Source: CAD feature listing. Evaluate the final solid. Frame: model axes, mm. A direction names the side the tool comes from. Coordinates: 2 decimals unless noted, no trailing zeros. Write each loop counter-clockwise with the first axis right and the second up, starting at its lowest first coordinate (ties: lowest second). Pieces come first, ordered by that corner, then holes. Notation, with made-up numbers: M 87,-1 L 104,-1 A19 ccw 104,12 Z; hole C 79,-3.75 d7. An arc over 180 degrees is marked long. One line per item, written item: value. Start each with the question number.
Item 1: Pin query (flat end, axial travel): P1, Ø3, axis at x = 0, z = 0, coming from the +Y side; P2, Ø2, axis at x = 9.5, z = 2, coming from the +Y side; P3, Ø1.5, axis at y = 1.5, z = -1, coming from the -X side; P4, Ø4, axis at x = -0.5, z = 0, coming from the +Y side. Return the tip coordinate at first contact, or that it passes through.
Item 2: Set-up query: faces 1 (the flat face through (2, 3.9, 2)), 2 (the flat face through (-1, 1, 1)), 3 (the cylindrical face through (-0.5, 2.7, 2.4)). Return all of +Z, -Z, +X, -X, +Y, -Y with unobstructed straight access to the full face (end or side cutting, diameter ignored); none if empty.
Item 3: Cut plane A-A, the plane y = 0.8. State how many separate pieces and enclosed holes the cut face has, then the cut area to 3 significant figures.
Item 4: Cut plane C-C, the plane z = 1.75. Output: boundary loops of the cut face in (x, y).
Item 5: Cut plane B-B, the plane x = 4.5. Output: boundary loops of the cut face in (y, z), then the cut area to 3 significant figures.
Item 6: Ray query, L1, parallel to Z at x = 0, y = 1.2; L2, parallel to Z at x = 15.2, y = 0.6; L3, parallel to X at y = 2.3, z = 0. Return the intervals inside material, ascending. Write a range as from..to.
Item 7: Mould query, pull axis X, two halves, no side actions, for faces 4 (the flat face through (10, 1.4, 1)), 5 (the flat face through (1, 1.5, -1)), 6 (the cylindrical face through (17.2, 0.7, 0)). Classes: released by +X, released by -X, zero draft, split by the parting line, or undercut.
```python
from build123d import *

# Parameters (mm, degrees)
SKETCH1_R           = 0.5
BOSS_EXTRUDE1_DEPTH = 1.4
SKETCH2_R           = 2.35
CUT_EXTRUDE1_DEPTH  = 1
SKETCH3_R           = 3.5
SKETCH3_R_2         = 2.45
BOSS_EXTRUDE2_DEPTH = 2.5
SKETCH4_R           = 1.2
CUT_EXTRUDE2_DEPTH  = 2.4
SKETCH5_R           = 2.45
SKETCH5_R_2         = 1.2
BOSS_EXTRUDE3_DEPTH = 0.1
SKETCH6_W           = 35.735260114
SKETCH6_H           = 17.672039004
CUT_EXTRUDE4_DEPTH  = 4.9
CUT_EXTRUDE5_DEPTH  = 4.9


with BuildPart() as part:
    # Sketch1 → Boss-Extrude1 (new body)
    with BuildSketch(Plane(origin=(0, 0, 0), x_dir=(1, 0, 0), z_dir=(0, 1, 0))):
        with BuildLine():
            Line((-15.2, 2), (-2, 2.95))
            Line((-2, 2.95), (-2, 6.35))
            ThreePointArc((-2, 6.35), (0, 8.35), (2, 6.35))
            Line((2, 6.35), (2, 3.5))
            Line((2, 3.5), (15.2, 2))
            ThreePointArc((15.2, 2), (17.2, 0), (15.2, -2))
            Line((15.2, -2), (2, -3.5))
            Line((2, -3.5), (2, -6.35))
            ThreePointArc((2, -6.35), (0, -8.35), (-2, -6.35))
            Line((-2, -6.35), (-2, -2.95))
            Line((-2, -2.95), (-15.2, -2))
            ThreePointArc((-15.2, -2), (-17.2, 0), (-15.2, 2))
        make_face()
        with Locations((0, 6.35)):
            Circle(SKETCH1_R, mode=Mode.SUBTRACT)
        with Locations((0, 4.55)):
            Circle(SKETCH1_R, mode=Mode.SUBTRACT)
        with Locations((0, -4.55)):
            Circle(SKETCH1_R, mode=Mode.SUBTRACT)
        with Locations((0, -6.35)):
            Circle(SKETCH1_R, mode=Mode.SUBTRACT)
        with Locations((-15.2, 0)):
            Circle(SKETCH1_R, mode=Mode.SUBTRACT)
        with Locations((15.2, 0)):
            Circle(SKETCH1_R, mode=Mode.SUBTRACT)
        with Locations((-13.4, 0)):
            Circle(SKETCH1_R, mode=Mode.SUBTRACT)
        with Locations((-11.6, 0)):
            Circle(SKETCH1_R, mode=Mode.SUBTRACT)
        with Locations((-9.8, 0)):
            Circle(SKETCH1_R, mode=Mode.SUBTRACT)
        with Locations((-8, 0)):
            Circle(SKETCH1_R, mode=Mode.SUBTRACT)
        with Locations((-6.2, 0)):
            Circle(SKETCH1_R, mode=Mode.SUBTRACT)
        with Locations((-4.4, 0)):
            Circle(SKETCH1_R, mode=Mode.SUBTRACT)
        with Locations((13.4, 0)):
            Circle(SKETCH1_R, mode=Mode.SUBTRACT)
        with Locations((11.6, 0)):
            Circle(SKETCH1_R, mode=Mode.SUBTRACT)
        with Locations((9.8, 0)):
            Circle(SKETCH1_R, mode=Mode.SUBTRACT)
        with Locations((8, 0)):
            Circle(SKETCH1_R, mode=Mode.SUBTRACT)
        with Locations((6.2, 0)):
            Circle(SKETCH1_R, mode=Mode.SUBTRACT)
        with Locations((4.4, 0)):
            Circle(SKETCH1_R, mode=Mode.SUBTRACT)
    extrude(amount=BOSS_EXTRUDE1_DEPTH)

    # Sketch2 → Cut-Extrude1 (cut)
    with BuildSketch(Plane.XZ):
        Circle(SKETCH2_R)
    extrude(amount=-CUT_EXTRUDE1_DEPTH, mode=Mode.SUBTRACT)

    # Sketch3 → Boss-Extrude2 (add)
    with BuildSketch(Plane(origin=(0, 1.4, 0), x_dir=(1, 0, 0), z_dir=(0, 1, 0))):
        Circle(SKETCH3_R)
        Circle(SKETCH3_R_2, mode=Mode.SUBTRACT)
    extrude(amount=BOSS_EXTRUDE2_DEPTH)

    # Sketch4 → Cut-Extrude2 (cut, through all)
    with BuildSketch(Plane(origin=(0, 1.4, 0), x_dir=(1, 0, 0), z_dir=(0, 1, 0))):
        Circle(SKETCH4_R)
    extrude(amount=-CUT_EXTRUDE2_DEPTH, mode=Mode.SUBTRACT)

    # Sketch5 → Boss-Extrude3 (add)
    with BuildSketch(Plane(origin=(0, 1.4, 0), x_dir=(1, 0, 0), z_dir=(0, 1, 0))):
        Circle(SKETCH5_R)
        Circle(SKETCH5_R_2, mode=Mode.SUBTRACT)
    extrude(amount=BOSS_EXTRUDE3_DEPTH)

    # Sketch6 → Cut-Extrude4 (cut, through all)
    with BuildSketch(Plane.XZ):
        Rectangle(SKETCH6_W, SKETCH6_H)
        with BuildLine():
            Line((-1.868584713, -2.959457918), (-15.2, -2))
            ThreePointArc((-15.2, -2), (-17.2, 0), (-15.2, 2))
            Line((-15.2, 2), (-1.868584713, 2.959457918))
            ThreePointArc((-1.868584713, 2.959457918), (0, 3.5), (1.868584713, 2.959457918))
            Line((1.868584713, 2.959457918), (15.2, 2))
            ThreePointArc((15.2, 2), (17.2, 0), (15.2, -2))
            Line((15.2, -2), (1.868584713, -2.959457918))
            ThreePointArc((1.868584713, -2.959457918), (0, -3.5), (-1.868584713, -2.959457918))
        make_face(mode=Mode.SUBTRACT)
    extrude(amount=-CUT_EXTRUDE4_DEPTH, mode=Mode.SUBTRACT)

    # Sketch7 → Cut-Extrude5 (cut, through all)
    with BuildSketch(Plane.XZ):
        with BuildLine():
            Line((0, 3.5), (-17.731768104, 3.5))
            Line((-17.731768104, 3.5), (-17.731768104, -3.5))
            Line((-17.731768104, -3.5), (0, -3.5))
            ThreePointArc((0, -3.5), (-3.5, 0), (0, 3.5))
        make_face()
    extrude(amount=-CUT_EXTRUDE5_DEPTH, mode=Mode.SUBTRACT)


solid = part.part
```
From the geometry:
1. P1: stops at y = 1.5
1. P2: stops at y = 1.4
1. P3: stops at x = -3.49
1. P4: stops at y = 3.9
2. face 1: +Z, -Z, +X, -X, +Y
2. face 2: -Y
2. face 3: +Y
3. separate pieces: 1
3. enclosed holes: 8
3. area: 81.2 mm²
4. outline: M -3.03,0 L -1.57,0 L -1.57,1 L 1.57,1 L 1.57,0 L 16.17,0 L 16.17,1.4 L 3.03,1.4 L 3.03,3.9 L 1.71,3.9 L 1.71,1.5 L -1.71,1.5 L -1.71,3.9 L -3.03,3.9 Z
5. outline: M 0,-2.77 L 1.4,-2.77 L 1.4,-0.49 L 0,-0.49 Z; M 0,0.49 L 1.4,0.49 L 1.4,2.77 L 0,2.77 Z
5. area: 6.38 mm²
6. L1: z = -3.5..-1.2, 1.2..3.5
6. L2: z = -2..-0.5, 0.5..2
6. L3: x = -3.5..-2.45, 2.45..3.5
7. face 4: zero draft
7. face 5: undercut
7. face 6: released by +X
